```python
from build123d import *

# Parameters (mm, degrees)
SKETCH002_R      = 1.5
SKETCH002_R_2    = 11
EXTRUDE002_DEPTH = 10
SKETCH001_R      = 3
EXTRUDE001_DEPTH = 7
SKETCH_W         = 70
SKETCH_H         = 54
EXTRUDE_DEPTH    = 3


with BuildPart() as extrude002:
    # Sketch002 (on Face5 of Extrude) → Extrude002 (new body, symmetric)
    with BuildSketch(Plane(origin=(0, 0, 0), x_dir=(1, 0, 0), z_dir=(0, 0, -1))):
        with Locations((-28.85, 25.473994)):
            Circle(SKETCH002_R)
        with Locations((28.85, 25.473994)):
            Circle(SKETCH002_R)
        with Locations((-28.85, -23.726006)):
            Circle(SKETCH002_R)
        with Locations((29.35, -23.726006)):
            Circle(SKETCH002_R)
        with Locations((-14.675, 11.863003)):
            Circle(SKETCH002_R_2)
        with Locations((-14.675, -11.863003)):
            Circle(SKETCH002_R_2)
        with Locations((14.675, 11.863003)):
            Circle(SKETCH002_R_2)
        with Locations((14.675, -11.863003)):
            Circle(SKETCH002_R_2)
    extrude(amount=EXTRUDE002_DEPTH, both=True)


with BuildPart() as extrude001:
    # Sketch001 (on Extrude) → Extrude001 (new body)
    with BuildSketch(Plane.XY):
        with Locations((-28.85, 23.726006)):
            Circle(SKETCH001_R)
        with Locations((29.35, 23.726006)):
            Circle(SKETCH001_R)
        with Locations((-28.85, -25.473994)):
            Circle(SKETCH001_R)
        with Locations((28.85, -25.473994)):
            Circle(SKETCH001_R)
    extrude(amount=-EXTRUDE001_DEPTH)


with BuildPart() as cut:
    # Sketch → Extrude (new body)
    with BuildSketch(Plane.XY):
        Rectangle(SKETCH_W, SKETCH_H)
    extrude(amount=EXTRUDE_DEPTH)

    # Fusion: union Extrude001
    add(extrude001.part)

    # Cut: cut Extrude002
    add(extrude002.part, mode=Mode.SUBTRACT)


solid = cut.part
```
Build history of the part. All positions in model axes, mm. A direction names the side the tool comes from. Coordinates: 2 decimals unless noted, no trailing zeros. Order: outer loops, then holes, each group sorted by start corner. A loop starts at its lowest first (then second) coordinate and runs counter-clockwise, first axis right, second up.
Item 1: Drill centre lines: L1, parallel to X at y = -11, z = 0.25; L2, parallel to X at y = 15.5, z = 2.5; L3, parallel to Y at x = -8, z = 2.25. Where is each one in solid material? Low to high.
Filled in:
L1: x = -35 to -25.64, -3.71 to 3.71, 25.64 to 35
L2: x = -35 to -25.06, -4.29 to 4.29, 25.06 to 35
L3: y = -27 to -20.61, -3.12 to 3.12, 20.61 to 27
Item 2: Tool access for faces 1 (the flat face through (29, -28, 0)), 2 (the cylindrical face through (-16.11, -22.77, 1.48)), 3 (the cylindrical face through (31.71, -24.57, -3.45)): list every direction of +Z, -Z, +X, -X, +Y, -Y with a clear straight run to the whole face (end or side of a thin tool).
Filled in:
face 1: +Z, +X, -X, -Y
face 2: +Z, -Z
face 3: -Z
Item 3: Saw through at B-B on z = -5.5. List the corners of the cut face in (x, y), then the cut area to 3 significant figures.
Filled in:
outline: circle Ø6 at (-28.85, -25.47); circle Ø6 at (-28.85, 23.73); circle Ø6 at (28.85, -25.47); circle Ø6 at (29.35, 23.73); hole circle Ø3 at (-28.85, -25.47); hole circle Ø3 at (-28.85, 23.73); hole circle Ø3 at (28.85, -25.47); hole circle Ø3 at (29.35, 23.73)
area: 84.8 mm2
Item 4: Saw through at A-A on x = -28.85. State how many separate pieces and enclosed holes the cut face has, then the cut area to 3 significant figures.
Filled in:
separate pieces: 3
enclosed holes: 0
area: 186 mm2
Item 5: Drop flat-ended pins along their axis: pin 1 Ø2.5 at (x, y) = (29.35, 23.73) entering from +Z; pin 2 Ø2 at (x, y) = (-25.5, -17.5) entering from -Z; pin 3 Ø1.5 at (x, z) = (-13.5, 1) entering from -Y. Give the stop position or say it passes through.
Filled in:
pin 1: passes through
pin 2: stops at z = 0
pin 3: stops at y = -27
Item 6: Saw through at C-C on y = 14. List the corners of the cut face in (x, z).
Filled in:
outline: (-35, 0) - (-25.47, 0) - (-25.47, 3) - (-35, 3) - close; (-3.88, 0) - (3.88, 0) - (3.88, 3) - (-3.88, 3) - close; (25.47, 0) - (35, 0) - (35, 3) - (25.47, 3) - close
Item 7: Saw through at D-D on x = 13. List the corners of the cut face in (y, z), then the cut area to 3 significant figures.
Filled in:
outline: (-27, 0) - (-22.73, 0) - (-22.73, 3) - (-27, 3) - close; (-0.99, 0) - (0.99, 0) - (0.99, 3) - (-0.99, 3) - close; (22.73, 0) - (27, 0) - (27, 3) - (22.73, 3) - close
area: 31.5 mm2
Item 8: Mould opens along Y. For faces 4 (the flat face through (0, -27, 1)), 5 (the cylindrical face through (-16.107, 0.957, 1.479)), 6 (the flat face through (0, 0, 3)) say: released by +Y, released by -Y, zero draft, split by the parting line, or undercut.
Filled in:
face 4: released by -Y
face 5: undercut
face 6: zero draft
